```python
from build123d import *

# Parameters (mm, degrees)
PAD001_DEPTH  = 3
PAD_DEPTH     = 80
SKETCH002_R   = 4
POCKET_DEPTH  = 3.001
SKETCH003_R   = 6
SKETCH003_R_2 = 4
PAD002_DEPTH  = 1


with BuildPart() as body001:
    # Sketch001 → Pad001 (new body)
    with BuildSketch(Plane.YZ):
        with BuildLine():
            Line((79.823677, 0), (0, 0))
            Line((0, 0), (0, 79.823677))
            Line((0, 79.823677), (2.832004, 79.823677))
            Line((2.832004, 79.823677), (2.831928, 79.536726))
            ThreePointArc((2.831928, 79.536726), (3.237512, 77.490861), (4.393829, 75.755062))
            Line((4.393829, 75.755062), (75.39639, 4.499797))
            ThreePointArc((75.39639, 4.499797), (77.239452, 3.264747), (79.41524, 2.830951))
            Line((79.823677, 2.830951), (79.41524, 2.830951))
            Line((79.823677, 0), (79.823677, 2.830951))
        make_face()
    extrude(amount=PAD001_DEPTH)


with BuildPart() as body001_1:
    # Body001 placement: moved
    add(body001.part.moved(Location((57, 0, 0))))


with BuildPart() as body002:
    # Body002 base: copy of Body001
    add(body001_1.part)


with BuildPart() as body002_1:
    # Clone placement: moved
    add(body002.part.moved(Location((4, 0, 0))))


with BuildPart() as body002_2:
    # Body002 placement: moved
    add(body002_1.part.moved(Location((-41, 0, 0))))


with BuildPart() as body003:
    # Body003 base: copy of Body001
    add(body001_1.part)


with BuildPart() as body003_1:
    # Body003 placement: moved
    add(body003.part.moved(Location((19, 0, 0))))


with BuildPart() as body004:
    # Body004 base: copy of Body001
    add(body001_1.part)


with BuildPart() as body004_1:
    # Body004 placement: moved
    add(body004.part.moved(Location((-55, 0, 0))))


with BuildPart() as fusion:
    # Sketch → Pad (new body)
    with BuildSketch(Plane.YZ):
        Polygon((0, 0), (0, 80), (3, 80), (3, 3), (80, 3), (80, 0), align=None)
    extrude(amount=PAD_DEPTH)

    # Sketch002 (on Face3 of Pad) → Pocket (cut, through all)
    with BuildSketch(Plane.ZX.offset(3)):
        with Locations((68.267296, 68.324082)):
            Circle(SKETCH002_R)
        with Locations((68.267296, 11.675918)):
            Circle(SKETCH002_R)
        with Locations((68.267296, 42.377682)):
            Circle(SKETCH002_R)
    extrude(amount=-POCKET_DEPTH, mode=Mode.SUBTRACT)

    # Sketch003 (on Face10 of Pocket) → Pad002 (join)
    with BuildSketch(Plane.ZX.offset(3)):
        with Locations((68.267296, 42.377682)):
            Circle(SKETCH003_R)
        with Locations((68.267296, 42.377682)):
            Circle(SKETCH003_R_2, mode=Mode.SUBTRACT)
        with Locations((68.267296, 11.675918)):
            Circle(SKETCH003_R)
        with Locations((68.267296, 11.675918)):
            Circle(SKETCH003_R_2, mode=Mode.SUBTRACT)
        with Locations((68.267296, 68.324082)):
            Circle(SKETCH003_R)
        with Locations((68.267296, 68.324082)):
            Circle(SKETCH003_R_2, mode=Mode.SUBTRACT)
    extrude(amount=PAD002_DEPTH)

    # Fusion: union Body001, Body002, Body003, Body004
    add(body001_1.part)
    add(body002_2.part)
    add(body003_1.part)
    add(body004_1.part)


solid = fusion.part
```
CAD build for the part. Positions are in the model's coordinates, mm. A direction names the side the tool comes from. Round coordinates to 2 decimals unless told otherwise and drop trailing zeros. Loops run counter-clockwise (first coordinate to the right, second up) from the corner with the lowest first, then second, coordinate; pieces in that order, holes last. Notation, with made-up numbers: M -4.5,42 L 14.5,42 A25 cw 14.5,73 Z; hole C 43,-26.75 d4. An arc over 180 degrees is marked long. Return JSON: item names as keys, results as strings. Group by question number.
(1) Saw through at A-A, the plane x = 67. List the corners of the cut face in (y, z), and give its area (3 significant figures).
(2) Drop flat-ended pins along their axis: P1, Ø22.5, axis at y = 22, z = 53, coming from the -X side; P2, Ø3, axis at x = 60.5, z = 36, coming from the +Y side; P3, Ø9, axis at x = 42.38, z = 68.27, coming from the -Y side; P4, Ø12, axis at x = 10, z = 29, coming from the +Y side. Give the stop position or say it passes through.
(3) Saw through at D-D, the plane x = 25. List the corners of the cut face in (y, z).
(4) Mould opens along Z. For faces 4 (the flat face through (57, 24, 24)), 5 (the flat face through (48, 3, 42)), 6 (the flat face through (21.479, 39.398, 40.626)) say: +Z half, -Z half, draft (parallel to the pull), parting line (faces both ways), or undercut.
(5) Saw through at B-B, the plane y = 37. List the corners of the cut face in (x, z), and give its area (3 significant figures).
(6) Tool access for faces 1 (the cylindrical face through (42.641, 3.493, 62.273)), 2 (the flat face through (60, 24, 24)), 3 (the flat face through (2, 24, 24)): list every direction of +Z, -Z, +X, -X, +Y, -Y with a clear straight run to the whole face (end or side of a thin tool).
(7) Saw through at C-C, the plane z = 34.5. List the corners of the cut face in (x, y), and give its area (3 significant figures).
(8) Wall check: probe 1 along X at (y, z) = (10, 33); probe 2 along Y at (x, z) = (44, 51.5). Give the ranges that are in metal, low to high. Write a range as [from, to].
Answer list:
{
 "1": {"outline": "M 0,0 L 80,0 L 80,3 L 3,3 L 3,62.42 L 4,62.42 L 4,64.49 L 0,64.49 Z; M 0,72.04 L 4,72.04 L 4,74.12 L 3,74.12 L 3,80 L 0,80 Z", "area": "453 mm2"},
 "2": {"P1": "x = 2", "P2": "y = 45.42", "P3": "y = 0", "P4": "y = 54.29"},
 "3": {"outline": "M 0,0 L 80,0 L 80,3 L 3,3 L 3,80 L 0,80 Z"},
 "4": {"face 4": "draft", "face 5": "undercut", "face 6": "+Z half"},
 "5": {"outline": "M 0,0 L 80,0 L 80,3 L 79,3 L 79,43.03 L 76,43.03 L 76,3 L 60,3 L 60,43.03 L 57,43.03 L 57,3 L 23,3 L 23,43.03 L 20,43.03 L 20,3 L 5,3 L 5,43.03 L 2,43.03 L 2,3 L 0,3 Z", "area": "720 mm2"},
 "6": {"face 1": "+Y", "face 2": "+Z, +Y", "face 3": "+Z, -X, +Y"},
 "7": {"outline": "M 0,0 L 80,0 L 80,3 L 79,3 L 79,45.5 L 76,45.5 L 76,3 L 60,3 L 60,45.5 L 57,45.5 L 57,3 L 23,3 L 23,45.5 L 20,45.5 L 20,3 L 5,3 L 5,45.5 L 2,45.5 L 2,3 L 0,3 Z", "area": "750 mm2"},
 "8": {"probe 1": "[2, 5], [20, 23], [57, 60], [76, 79]", "probe 2": "[0, 3]"}
}
